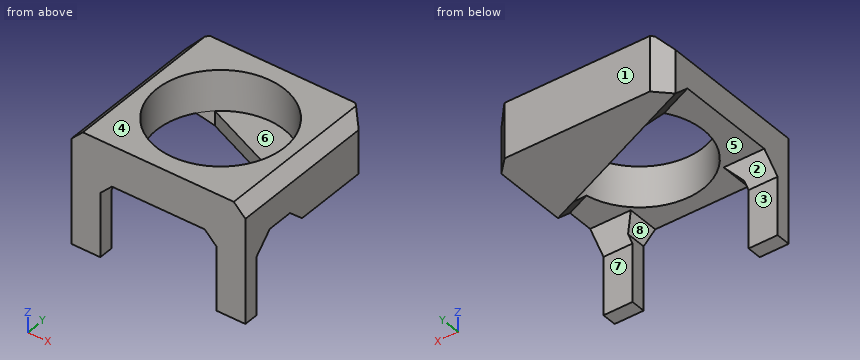
```python
from build123d import *

# Parameters (mm, degrees)
SKETCH1_R           = 11
BOSS_EXTRUDE1_DEPTH = 7
SKETCH2_W           = 5
SKETCH2_H           = 2.5
BOSS_EXTRUDE2_DEPTH = 13
CHAMFER1_SIZE       = 3
CHAMFER2_SIZE       = 2
CHAMFER3_SIZE       = 2
CHAMFER4_SIZE       = 2
BOSS_EXTRUDE4_DEPTH = 2.5
CHAMFER6_SIZE       = 2.5


with BuildPart() as part:
    # Sketch1 → Boss-Extrude1 (new body)
    with BuildSketch(Plane.XY):
        Polygon((-15, 11.5), (-12.5, 14), (12.5, 14), (15, 11.5), (15, -14), (-15, -14), align=None)
        Circle(SKETCH1_R, mode=Mode.SUBTRACT)
    extrude(amount=BOSS_EXTRUDE1_DEPTH)

    # Sketch2 → Boss-Extrude2 (add)
    with BuildSketch(Plane(origin=(0, 0, 0), x_dir=(-1, 0, 0), z_dir=(0, 0, -1))):
        with Locations((-12.5, -12.75)):
            Rectangle(SKETCH2_W, SKETCH2_H)
        with Locations((12.5, -12.75)):
            Rectangle(SKETCH2_W, SKETCH2_H)
    extrude(amount=BOSS_EXTRUDE2_DEPTH)

    # Chamfer1
    chamfer1_edges = [part.edges().sort_by_distance(p)[0] for p in [
        (-12.5, -11.5, 0),
        (12.5, -11.5, 0),
    ]]
    chamfer(chamfer1_edges, length=CHAMFER1_SIZE)

    # Chamfer2
    chamfer2_edges = [part.edges().sort_by_distance(p)[0] for p in [
        (-10, -11.25, 0),
        (10, -11.25, 0),
    ]]
    chamfer(chamfer2_edges, length=CHAMFER2_SIZE)

    # Chamfer3
    chamfer3_edges = [part.edges().sort_by_distance(p)[0] for p in [
        (15, -1.25, 7),
    ]]
    chamfer(chamfer3_edges, length=CHAMFER3_SIZE)

    # Chamfer4
    chamfer4_edges = [part.edges().sort_by_distance(p)[0] for p in [
        (-15, -1.25, 7),
    ]]
    chamfer(chamfer4_edges, length=CHAMFER4_SIZE)

    # Sketch4 → Boss-Extrude4 (add)
    with BuildSketch(Plane(origin=(0, 0, 0), x_dir=(-1, 0, 0), z_dir=(0, 0, -1))):
        Polygon((-15, -1.25), (15, 11.5), (12.5, 14), (-12.5, 14), (-15, 11.5), align=None)
    extrude(amount=BOSS_EXTRUDE4_DEPTH)

    # Chamfer6
    # the kernel refuses this chamfer: 2.5 mm, written as the material it adds along each edge
    with BuildSketch(Plane(origin=(20.916998416, -3.764724327, 0), x_dir=(0.01075475478430782, 0.02530530537484193, -0.9996219169112968), z_dir=(-0.9203309184584746, 0.39114064034485174, 0))) as chamfer6_piece_1_section:
        Polygon((CHAMFER6_SIZE * 0.999621916911, CHAMFER6_SIZE * 0.0274958766106), (-CHAMFER6_SIZE * 0.0274958766106, CHAMFER6_SIZE * 0.999621916911), (0, 0), align=None)
    chamfer6_piece_1 = extrude(amount=17.214861222, mode=Mode.PRIVATE)
    chamfer6_piece_1 = chamfer6_piece_1 - Plane(origin=(0, 0, -0.830769879), x_dir=(1, 0, 0), z_dir=(0, 0, -1)) * Cylinder(11, 45, mode=Mode.PRIVATE)
    chamfer6_piece_1 = split(chamfer6_piece_1, bisect_by=Plane(origin=(15, -1.305255327, -0.830769879), z_dir=(-1, 0, 0)), keep=Keep.TOP, mode=Mode.PRIVATE)
    add(chamfer6_piece_1)
    with BuildSketch(Plane(origin=(-1.383846422, 5.71313473, 0), x_dir=(0.010754754784307773, 0.025305305374841817, -0.9996219169112968), z_dir=(-0.9203309184584746, 0.39114064034485174, 0))) as chamfer6_piece_2_section:
        Polygon((CHAMFER6_SIZE * 0.999621916911, CHAMFER6_SIZE * 0.0274958766106), (-CHAMFER6_SIZE * 0.0274958766106, CHAMFER6_SIZE * 0.999621916911), (0, 0), align=None)
    chamfer6_piece_2 = extrude(amount=21.224052785, mode=Mode.PRIVATE)
    chamfer6_piece_2 = chamfer6_piece_2 - Plane(origin=(0, 0, -0.851096237), x_dir=(1, 0, 0), z_dir=(0, 0, -1)) * Cylinder(11, 53, mode=Mode.PRIVATE)
    chamfer6_piece_2 = split(chamfer6_piece_2, bisect_by=Plane(origin=(-15, 9.126408424, -0.851096237), z_dir=(1, 0, 0)), keep=Keep.TOP, mode=Mode.PRIVATE)
    add(chamfer6_piece_2)


solid = part.part
```
Source: CAD feature listing. Evaluate the final solid. Frame: model axes, mm. Face numbers are marked on the shaded views. A direction names the side the tool comes from. Round coordinates to 2 decimals unless told otherwise and drop trailing zeros. Loops run counter-clockwise (first coordinate to the right, second up) from the corner with the lowest first, then second, coordinate; pieces in that order, holes last.
1. Section query A-A on z = -6. Output: boundary loops of the cut face in (x, y).
2. Section query D-D on y = -4.75. Output: boundary loops of the cut face in (x, z).
3. Section query B-B on z = 5.5. Output: boundary loops of the cut face in (x, y).
4. Mould query, pull axis Y, two halves, no side actions, for the marked faces 6, 7 and 8. Classes: released by +Y, released by -Y, zero draft, split by the parting line, or undercut.
5. Contact query for flat-ended pins moving along their axis: pin 1 (5.5 mm diameter, centred on x = 13, z = -9.5, fed in from +Y); pin 2 (7.5 mm diameter, centred on x = 4.5, y = 7.5, fed in from -Z); pin 3 (3 mm diameter, centred on x = 0, y = 6, fed in from +Z). Output: stop coordinate, or through.
6. Ray query, L1, parallel to X at y = 0, z = 4.25; L2, parallel to Y at x = 0, z = 2.5; L3, parallel to X at y = -12, z = -6.25. Return the intervals inside material, ascending.
7. Access query for the marked faces 1, 2, 3, 4 and 5. Directions: +Z, -Z, +X, -X, +Y, -Y. A direction counts if a zero-diameter tool reaches every point of the face in a straight line with its end or side. Return the directions, or none.
8. Section query C-C on x = 9. Output: boundary loops of the cut face in (y, z), and give its area (3 significant figures).
Answers below:
1. outline: (-15, -14) - (-10, -14) - (-10, -11.5) - (-15, -11.5) - close; (10, -14) - (15, -14) - (15, -11.5) - (10, -11.5) - close
2. outline: (-15, 0) - (-9.92, 0) - (-9.92, 7) - (-13, 7) - (-15, 5) - close; (9.92, 0) - (15, 0) - (15, 5) - (13, 7) - (9.92, 7) - close
3. outline: (-14.5, -14) - (14.5, -14) - (14.5, 12) - (12.5, 14) - (-12.5, 14) - (-14.5, 12) - close; hole circle Ø22 at (0, 0)
4. face 6: undercut
4. face 7: released by +Y
4. face 8: zero draft
5. pin 1: stops at y = -11.5
5. pin 2: stops at z = -2.5
5. pin 3: stops at z = 0
6. L1: x = -15 to -11, 11 to 15
6. L2: y = -14 to -11, 11 to 14
6. L3: x = -15 to -10, 10 to 15
7. face 1: +Z, -Z, +X, -X, +Y
7. face 2: -Z, +X, -X
7. face 3: -Z, +X, -X, +Y
7. face 4: +Z, +X, -X, +Y, -Y
7. face 5: -Z
8. outline: (-14, -1) - (-9.5, -1) - (-8.5, 0) - (-6.32, 0) - (-6.32, 7) - (-14, 7) - close; (1.3, -2.5) - (14, -2.5) - (14, 7) - (6.32, 7) - (6.32, 0) - (1.3, 0) - close
8. area: 144 mm2
